```python
from build123d import *

# Parameters (mm, degrees)
SKETCH1_W             = 12.7
SKETCH1_H             = 12.7
BOSS_EXTRUDE1_DEPTH   = 1.5875
F_2_CLEARANCE_HOLE1_D = 2.4384
CHAMFER1_SIZE         = 1.27


with BuildPart() as part:
    # Sketch1 → Boss-Extrude1 (new body)
    with BuildSketch(Plane(origin=(0, 0, 0), x_dir=(1, 0, 0), z_dir=(0, 1, 0))):
        Rectangle(SKETCH1_W, SKETCH1_H)
    extrude(amount=BOSS_EXTRUDE1_DEPTH)

    # #2 Clearance Hole1 (through all)
    with Locations(Plane(origin=(0, 1.5875, 0), x_dir=(1, 0, 0), z_dir=(0, 1, 0))):
        with Locations((-4.3053, 4.3053), (4.3053, 4.3053), (4.3053, -4.3053), (-4.3053, -4.3053)):
            Hole(F_2_CLEARANCE_HOLE1_D / 2)

    # Chamfer1
    chamfer1_edges = [part.edges().sort_by_distance(p)[0] for p in [
        (6.35, 0.79375, 6.35),
        (-6.35, 0.79375, 6.35),
        (-6.35, 0.79375, -6.35),
        (6.35, 0.79375, -6.35),
    ]]
    chamfer(chamfer1_edges, length=CHAMFER1_SIZE)


solid = part.part
```
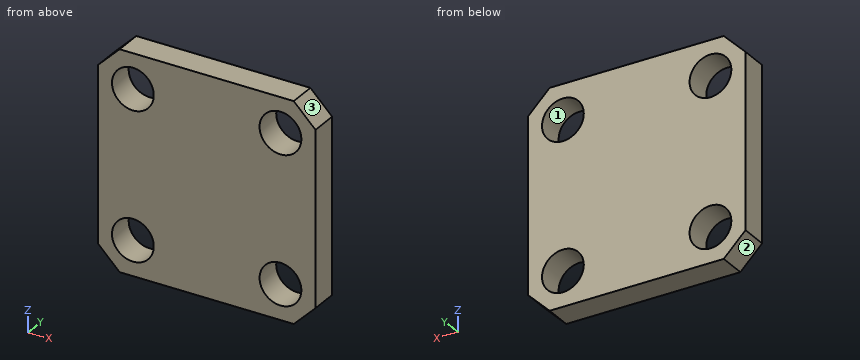
Build history of the part. All positions in model axes, mm. Face numbers are marked on the shaded views. Round coordinates to 2 decimals unless told otherwise and drop trailing zeros. Write each loop counter-clockwise with the first axis right and the second up, starting at its lowest first coordinate (ties: lowest second). Pieces come first, ordered by that corner, then holes.
1) Band-saw the part on B-B, the plane z = -4.75. List the corners of the cut face in (x, y).
2) Band-saw the part on C-C, the plane y = 0.55. List the corners of the cut face in (x, z).
3) Pin check, flat tip, straight feed: pin 1 (1.5 mm diameter, centred on x = 4.31, z = -4.31, fed in from -Y). Stop position of the tip, or through.
4) Band-saw the part on A-A, the plane x = -3.5. List the corners of the cut face in (y, z), and give its area (3 significant figures).
5) Band-saw the part on D-D, the plane x = 5.75. List the corners of the cut face in (y, z).
6) Drill centre lines: probe 1 along X at (y, z) = (0.4, 4.5); probe 2 along X at (y, z) = (0.7, 3.75). Where is each one in solid material? Low to high.
7) Mould opens along X. For the marked faces 1, 2 and 3 say: +X half, -X half, draft (parallel to the pull), parting line (faces both ways), or undercut.
Ans:
1. outline: (-6.35, 0) - (-5.44, 0) - (-5.44, 1.59) - (-6.35, 1.59) - close; (-3.17, 0) - (3.17, 0) - (3.17, 1.59) - (-3.17, 1.59) - close; (5.44, 0) - (6.35, 0) - (6.35, 1.59) - (5.44, 1.59) - close
2. outline: (-6.35, -5.08) - (-5.08, -6.35) - (5.08, -6.35) - (6.35, -5.08) - (6.35, 5.08) - (5.08, 6.35) - (-5.08, 6.35) - (-6.35, 5.08) - close; hole circle Ø2.44 at (-4.31, -4.31); hole circle Ø2.44 at (-4.31, 4.31); hole circle Ø2.44 at (4.31, -4.31); hole circle Ø2.44 at (4.31, 4.31)
3. pin 1: passes through
4. outline: (0, -6.35) - (1.59, -6.35) - (1.59, -5.22) - (0, -5.22) - close; (0, -3.39) - (1.59, -3.39) - (1.59, 3.39) - (0, 3.39) - close; (0, 5.22) - (1.59, 5.22) - (1.59, 6.35) - (0, 6.35) - close
4. area: 14.3 mm2
5. outline: (0, -5.68) - (1.59, -5.68) - (1.59, 5.68) - (0, 5.68) - close
6. probe 1: x = -6.35 to -5.51, -3.1 to 3.1, 5.51 to 6.35
6. probe 2: x = -6.35 to -5.39, -3.22 to 3.22, 5.39 to 6.35
7. face 1: undercut
7. face 2: -X half
7. face 3: +X half
